Could you check a few things on this drawing? It's one solid part, dimensions in mm from its lowest x, y, z. A direction names the side the tool comes from. Round coordinates to 2 decimals unless told otherwise and drop trailing zeros. Write each loop counter-clockwise with the first axis right and the second up, starting at its lowest first coordinate (ties: lowest second). Pieces come first, ordered by that corner, then holes. Notation, with made-up numbers: (-10, 72.5) -> (41, 72.5) arc R22 ccw to (41, 95.5) -> close; hole circle Ø5 at (-11, 78.5). An arc over 180 degrees is marked (long way). Put each result on its own line as item: value. Start each with the question number.
1) I want a section at B-B, the plane x = 25. List the corners of the cut face in (y, z) for me.
2) Will these pins go through, and if not, where does the flat tip stop? P1, Ø8, axis at x = 51.5, z = 30.5, coming from the +Y side; P2, Ø22, axis at x = 34, y = 34.5, coming from the +Z side; P3, Ø5, axis at x = 39, z = 14.5, coming from the +Y side.
3) I want a section at A-A, the plane z = 13.5. List the corners of the cut face in (x, y) for me, then the cut area to 3 significant figures.
4) If I drill on line 1 along Y through (x, z) = (9.5, 36.5); line 2 along X through (y, z) = (37, 19.5), over which ranges is the centre line in solid material (lowest first)? Write a range as [from, to].
5) I want a section at C-C, the plane y = 9. List the corners of the cut face in (x, z) for me.
6) I want a section at D-D, the plane z = 25. List the corners of the cut face in (x, y) for me.
7) Which directions (+Z, -Z, +X, -X, +Y, -Y) give clear straight access to the entire face, cutting with the end or side of a thin tool? Please do the marked faces 1, 2 and 3.
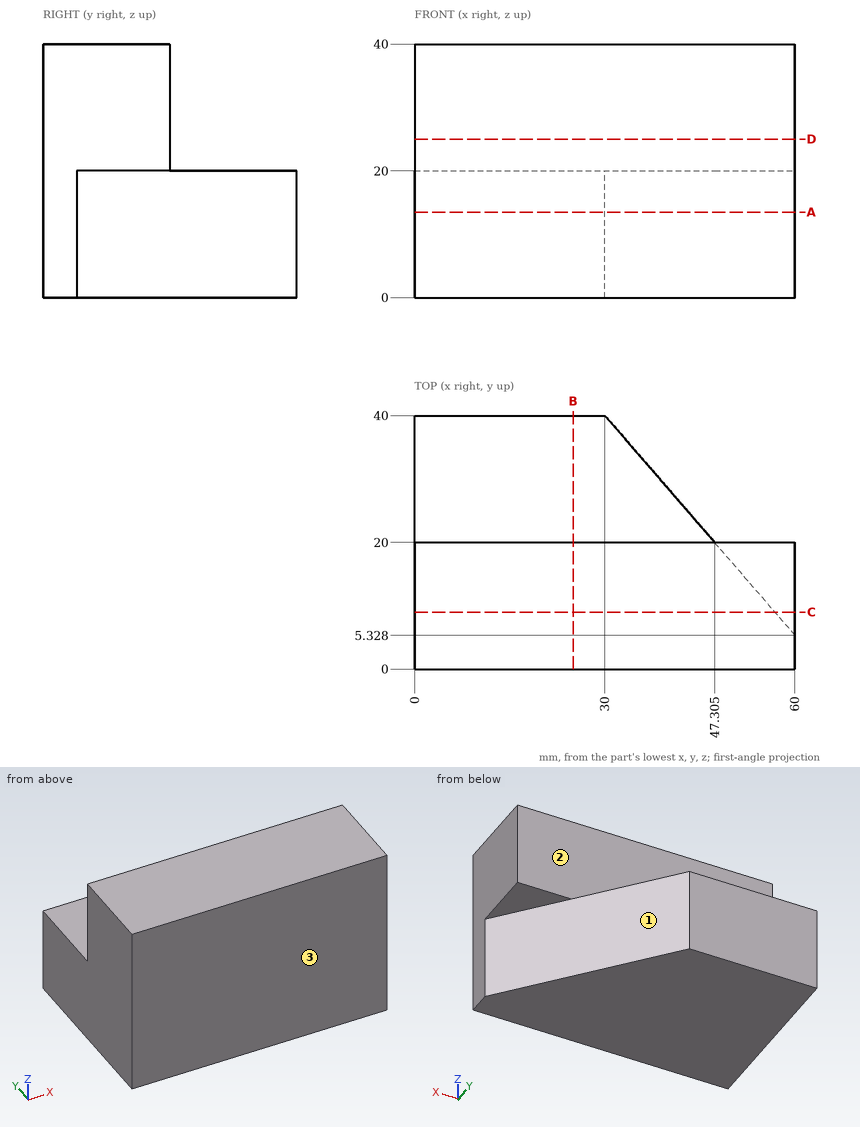
Findings:
1. outline: (0, 0) -> (40, 0) -> (40, 20) -> (20, 20) -> (20, 40) -> (0, 40) -> close
2. P1: stops at y = 20
2. P2: stops at z = 20
2. P3: stops at y = 32.49
3. outline: (0, 0) -> (60, 0) -> (60, 5.33) -> (30, 40) -> (0, 40) -> close
3. area: 1,880 mm2
4. line 1: y = [0, 20]
4. line 2: x = [0, 32.6]
5. outline: (0, 0) -> (56.82, 0) -> (56.82, 20) -> (60, 20) -> (60, 40) -> (0, 40) -> close
6. outline: (0, 0) -> (60, 0) -> (60, 20) -> (0, 20) -> close
7. face 1: -Z, +X, +Y
7. face 2: +Z, +X, -X, +Y
7. face 3: +Z, -Z, +X, -X, -Y
